Build history of the part. All positions in model axes, mm. A direction names the side the tool comes from. Round coordinates to 2 decimals unless told otherwise and drop trailing zeros. Order: outer loops, then holes, each group sorted by start corner. A loop starts at its lowest first (then second) coordinate and runs counter-clockwise, first axis right, second up. Notation, with made-up numbers: M 78.5,13 L 91.5,13 A16 cw 91.5,32 Z; hole C -27.75,49 d3. An arc over 180 degrees is marked long. One line per question, with ' | ' between items. Start each with the question number.
Autodesk Inventor part; units mm, degrees
ref_plane "Work Plane3" through (0, 5, 0) normal (0, 1, 0) x (-1, 0, 0)
ref_plane "Work Plane4" through (0, -5, 0) normal (0, 1, 0) x (-1, 0, 0)
ref_plane "Work Plane5" through (-5, 0, 0) normal (-1, 0, 0) x (0, -1, 0)
sketch "Sketch1" plane through (0, 0, 0) normal (0, 0, 1) x (1, 0, 0)
  circle A0 centre (0, 0) radius 5
  dimension "d0" = 10
extrude "Extrusion1" add sketch "Sketch1" along normal blind 10 and the other way blind 28.1
sketch "Sketch2" plane through (0, 0, 10) normal (0, 0, 1) x (1, 0, 0)
  line L0 (-2.7, -1.7996) -> (2.7, -1.7996)
  line L1 (2.7, -1.7996) -> (2.7, 1.7996)
  line L2 (2.7, 1.7996) -> (-2.7, 1.7996)
  line L3 (-2.7, 1.7996) -> (-2.7, -1.7996)
  line L4 (-2.7, -1.7996) -> (2.7, 1.7996) construction
  line L5 (2.7, -1.7996) -> (-2.7, 1.7996) construction
  point P0 (0, 0)
  dimension "d3" = 5.4
  dimension "d4" = 3.5992
extrude "Extrusion2" cut sketch "Sketch2" against normal blind 7.8994
ref_plane "Work Plane1" through (0, 0, 0) normal (0, 1, 0) x (0, 0, 1)
ref_plane "Work Plane2" through (0, 0, 0) normal (-1, 0, 0) x (0, 0, 1)
sketch "Sketch3" plane through (0, 0, 0) normal (0, 1, 0) x (0, 0, 1)
  point P0 (0, 0)
ref_plane "Work Plane3" through (0, 5, 0) normal (0, 1, 0) x (-1, 0, 0)
ref_plane "Work Plane4" through (0, -5, 0) normal (0, 1, 0) x (-1, 0, 0)
ref_plane "Work Plane5" through (-5, 0, 0) normal (-1, 0, 0) x (0, -1, 0)
ref_plane "Work Plane6" through (5, 0, 0) normal (-1, 0, 0) x (0, -1, 0)
sketch "Sketch4" plane through (0, 5, 0) normal (0, 1, 0) x (-1, 0, 0)
  point P0 (0, 0)
sketch "Sketch5" plane through (0, 5, 0) normal (0, 1, 0) x (-1, 0, 0)
  line L0 (5, 10) -> (-5, 10)
  line L1 (-2.5348, 10) -> (2.5348, 10)
  line L2 (2.5348, 10) -> (2.5348, -28.0998)
  line L3 (2.5348, -28.0998) -> (-2.5348, -28.0998)
  line L4 (-2.5348, -28.0998) -> (-2.5348, 10)
  point P0 (0, 0)
sketch "Sketch6" plane through (5, 0, 0) normal (-1, 0, 0) x (0, -1, 0)
  line L0 (-2.5348, 10) -> (2.5348, 10)
  line L1 (2.5348, 10) -> (2.5348, -28.0998)
  line L2 (2.5348, -28.0998) -> (-2.5348, -28.0998)
  line L3 (-2.5348, -28.0998) -> (-2.5348, 10)
  point P0 (0, 0)
sketch "Sketch7" plane through (0, -5, 0) normal (0, 1, 0) x (-1, 0, 0)
  point P0 (0, 0)
sketch "Sketch8" plane through (0, -5, 0) normal (0, 1, 0) x (-1, 0, 0)
  line L0 (-2.5348, 10) -> (2.5348, 10)
  line L1 (2.5348, 10) -> (2.5348, -28.0998)
  line L2 (2.5348, -28.0998) -> (-2.5348, -28.0998)
  line L3 (-2.5348, -28.0998) -> (-2.5348, 10)
  point P0 (0, 0)
sketch "Sketch9" plane through (0, -5, 0) normal (0, 1, 0) x (-1, 0, 0)
  point P0 (0, 0)
sketch "Sketch10" plane through (-5, 0, 0) normal (-1, 0, 0) x (0, -1, 0)
  line L0 (5, 10) -> (-5, 10)
  line L1 (-2.5422, 10) -> (2.5378, 10)
  line L2 (2.5378, 10) -> (2.5378, -28.1)
  line L3 (2.5378, -28.1) -> (-2.5422, -28.1)
  line L4 (-2.5422, -28.1) -> (-2.5422, 10)
  point P0 (0, 0)
  dimension "d9" = 5.08
  dimension "d10" = 38.1
extrude "Extrusion3" add sketch "Sketch5" along normal blind 36.83 and the other way blind 1.27
extrude "Extrusion4" add sketch "Sketch6" along normal blind 1.27 and the other way blind 36.83
extrude "Extrusion5" add sketch "Sketch10" along normal blind 36.83 and the other way blind 1.27
extrude "Extrusion6" add sketch "Sketch8" along normal blind 1.27 and the other way blind 36.83
properties part number "windmill"
Item 1: Cut at B-B on z = -24. Write the cut outline in (x, y).
Item 2: Cut at C-C on y = -27. Write the cut outline in (x, z).
Item 3: Flat gauge pins, fed straight in: pin 1 (11.5 mm diameter, centred on x = 25, z = -5.5, fed in from +Y); pin 2 (11.5 mm diameter, centred on y = -14.5, z = -12.5, fed in from -X); pin 3 (5 mm diameter, centred on x = 28.5, z = -13.5, fed in from -Y). Where does each tip first touch, or does it go through?
Item 4: Wall check: line 1 along X through (y, z) = (32.5, -17); line 2 along X through (y, z) = (-3, -13.5). Give the ranges that are in metal, low to high. Write a range as [from, to].
Item 5: Two-plate mould, pull along Y, no slides. Class faces 6 (the face through (-23, 2.542, -9)), 7 (the face through (0, 23, -28.1)), 8 (the face through (0, 0, 2.101)), 9 (the face through (-2.7, 0, 6)): +Y half, -Y half, draft (parallel to the pull), parting line (faces both ways), or undercut.
Item 6: Tool access for faces 1 (the face through (23, 2.535, -9)), 2 (the face through (23, -2.535, -9)), 3 (the face through (0, 1.8, 6)), 4 (the face through (-23, -2.538, -9)), 5 (the face through (-2.535, 23, -9)): list every direction of +Z, -Z, +X, -X, +Y, -Y with a clear straight run to the whole face (end or side of a thin tool).
Item 7: Cut at A-A on z = 5. Write the cut outline in (x, y).
Results found:
1) outline: M -41.83,-2.54 L -4.31,-2.54 A5 ccw -2.53,-4.31 L -2.53,-41.83 L 2.53,-41.83 L 2.53,-4.31 A5 ccw 4.31,-2.53 L 41.83,-2.53 L 41.83,2.53 L 4.31,2.53 A5 ccw 2.53,4.31 L 2.53,41.83 L -2.53,41.83 L -2.53,4.31 A5 ccw -4.31,2.54 L -41.83,2.54 Z
2) outline: M -2.53,-28.1 L 2.53,-28.1 L 2.53,10 L -2.53,10 Z
3) pin 1: stops at y = 2.53 | pin 2: stops at x = -2.53 | pin 3: stops at y = -2.53
4) line 1: x = [-2.53, 2.53] | line 2: x = [-4, 4]
5) face 6: +Y half | face 7: draft | face 8: undercut | face 9: undercut
6) face 1: +Z, -Z, +X, +Y | face 2: +Z, -Z, +X, -Y | face 3: +Z | face 4: +Z, -Z, -X, -Y | face 5: +Z, -Z, -X, +Y
7) outline: M -41.83,-2.54 L -4.31,-2.54 A5 ccw -2.53,-4.31 L -2.53,-41.83 L 2.53,-41.83 L 2.53,-4.31 A5 ccw 4.31,-2.53 L 41.83,-2.53 L 41.83,2.53 L 4.31,2.53 A5 ccw 2.53,4.31 L 2.53,41.83 L -2.53,41.83 L -2.53,4.31 A5 ccw -4.31,2.54 L -41.83,2.54 Z; hole M -2.7,-1.8 L 2.7,-1.8 L 2.7,1.8 L -2.7,1.8 Z
